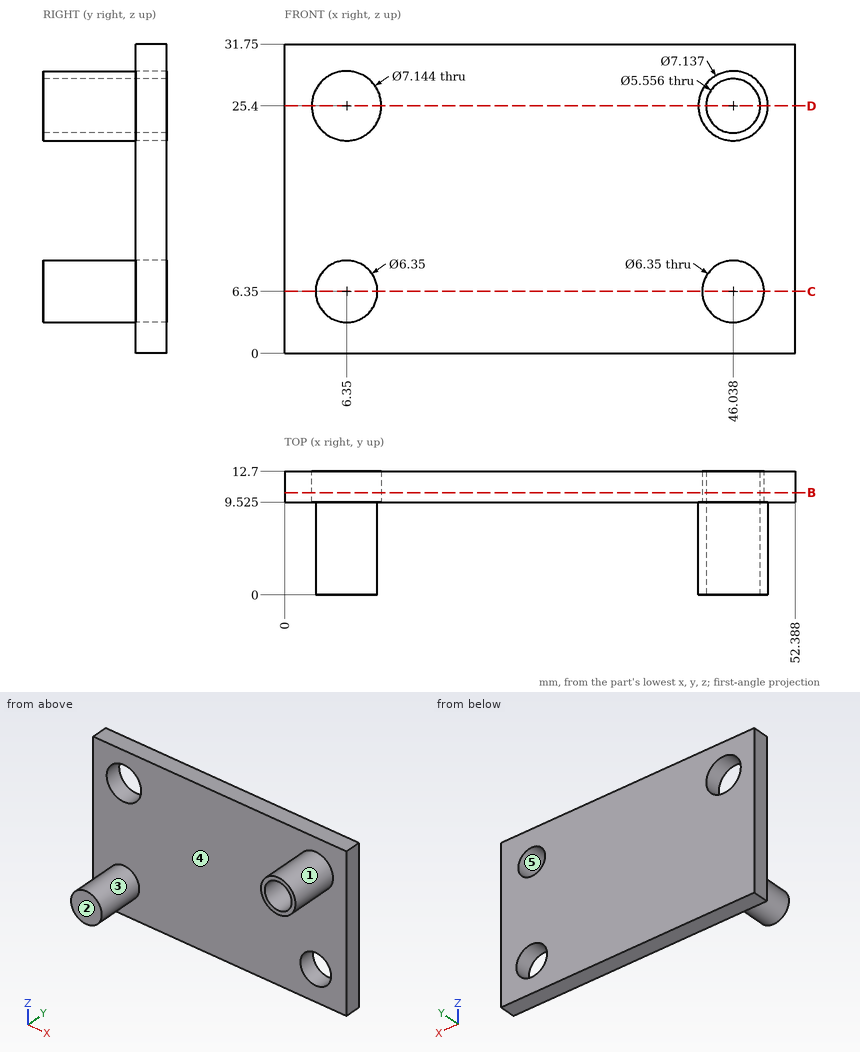
Here's the drawing with two shaded views (mm, measured from the low corner). I have some questions. A direction names the side the tool comes from. Give positions to 0.01 mm unless a question says otherwise; leave off trailing zeros. Order: outer loops, then holes, each group sorted by start corner. A loop starts at its lowest first (then second) coordinate and runs counter-clockwise, first axis right, second up. Notation, with made-up numbers: M 48.25,-3 L 101.25,-3 A37 cw 101.25,34 Z; hole C 5.5,88.25 d7. An arc over 180 degrees is marked long. Answer as a JSON object with one key per item and string values. Group by question number.
1) I'm going to push flat-ended pins straight in: pin 1 Ø5 at (x, z) = (46.04, 25.4) entering from +Y; pin 2 Ø2 at (y, z) = (11, 18) entering from -X; pin 3 Ø6 at (x, y) = (46.5, 1.5) entering from +Z; pin 4 Ø5 at (x, z) = (27.5, 7) entering from -Y (1 decimal). Where does each tip first touch, or does it pass through?
2) Suppose I cut it at B-B, the plane y = 10.5. Count the separate pieces of the cut face and the enclosed holes in it, plus the area to 3 significant figures.
3) Suppose I cut it at D-D, the plane z = 25.4. Write out the boundary of the cut face in (x, y) (1 decimal).
4) On a 3-axis mill with a long thin cutter (end or side, diameter ignored), from which of +Z, -Z, +X, -X, +Y, -Y can I reach the whole of each face in a straight line? I mean the marked faces 1 and 2. Say none if no direction works.
5) Please list where these lines run through material, in increasing order: L1, parallel to Y at x = 48.5, z = 20.5 (1 decimal); L2, parallel to Z at x = 6.35, y = 10.8; L3, parallel to X at y = 1.25, z = 26.5 (1 decimal). Write a range as [from, to].
6) We'd pull the mould along Z, two halves only. Please class the marked faces 3, 4 and 5: pulls with the +Z half, pulls with the -Z half, needs draft (parallel to the pull), parting line crosses it, or undercut.
7) Suppose I cut it at C-C, the plane z = 6.35. Write out the boundary of the cut face in (x, y) (1 decimal).
Results found:
{
 "1": {"pin 1": "through", "pin 2": "x = 0", "pin 3": "z = 28.97", "pin 4": "y = 9.5"},
 "2": {"separate pieces": "1", "enclosed holes": "3", "area": "1,570 mm²"},
 "3": {"outline": "M 0,9.5 L 2.8,9.5 L 2.8,12.7 L 0,12.7 Z; M 9.9,9.5 L 42.5,9.5 L 42.5,0 L 43.3,0 L 43.3,12.7 L 9.9,12.7 Z; M 48.8,0 L 49.6,0 L 49.6,9.5 L 52.4,9.5 L 52.4,12.7 L 48.8,12.7 Z"},
 "4": {"face 1": "-Y", "face 2": "+Z, -Z, +X, -X, -Y"},
 "5": {"L1": "[9.5, 12.7]", "L2": "[0, 21.83], [28.97, 31.75]", "L3": "[42.6, 43.5], [48.6, 49.4]"},
 "6": {"face 3": "parting line crosses it", "face 4": "needs draft", "face 5": "undercut"},
 "7": {"outline": "M 0,9.5 L 3.2,9.5 L 3.2,0 L 9.5,0 L 9.5,9.5 L 42.9,9.5 L 42.9,12.7 L 0,12.7 Z; M 49.2,9.5 L 52.4,9.5 L 52.4,12.7 L 49.2,12.7 Z"}
}
